from build123d import *

# Parameters (mm, degrees)
CROQUIS1_W              = 72
CROQUIS1_H              = 180
CROQUIS1_R              = 1.6
SALIENTE_EXTRUIR1_DEPTH = 4
CROQUIS2_R              = 3
CORTAR_EXTRUIR1_DEPTH   = 1.65
CROQUIS3_W              = 5
CROQUIS3_H              = 10
SALIENTE_EXTRUIR2_DEPTH = 10
CORTAR_EXTRUIR2_REACH   = 263.951
CROQUIS4_R              = 1.5
CROQUIS4_3_R            = 1.5
CORTAR_EXTRUIR3_DEPTH   = 1.65
REDONDEO2_R             = 10
CORTAR_EXTRUIR4_REACH   = 262.458
CROQUIS6_W              = 11.3
CROQUIS6_H              = 119.12
CORTAR_EXTRUIR5_DEPTH   = 4
REDONDEO3_R             = 3


with BuildPart() as part:
    # Croquis1 → Saliente-Extruir1 (new body)
    with BuildSketch(Plane.XY):
        with Locations((26, 162.773389683)):
            Rectangle(CROQUIS1_W, CROQUIS1_H)
        with Locations((-1.52, 76.973389683)):
            Circle(CROQUIS1_R, mode=Mode.SUBTRACT)
        with Locations((5.52, 83.573389683)):
            Circle(CROQUIS1_R, mode=Mode.SUBTRACT)
        with Locations((-1.52, 241.973389683)):
            Circle(CROQUIS1_R, mode=Mode.SUBTRACT)
        with Locations((5.52, 248.573389683)):
            Circle(CROQUIS1_R, mode=Mode.SUBTRACT)
    extrude(amount=SALIENTE_EXTRUIR1_DEPTH)

    # Croquis2 → Cortar-Extruir1 (cut)
    with BuildSketch(Plane.XY.offset(4)):
        with Locations((-1.52, 76.973389683)):
            Circle(CROQUIS2_R)
        with Locations((5.52, 83.573389683)):
            Circle(CROQUIS2_R)
        with Locations((-1.52, 241.973389683)):
            Circle(CROQUIS2_R)
        with Locations((5.52, 248.573389683)):
            Circle(CROQUIS2_R)
    extrude(amount=-CORTAR_EXTRUIR1_DEPTH, mode=Mode.SUBTRACT)

    # Croquis3 → Saliente-Extruir2 (add)
    with BuildSketch(Plane(origin=(0, 0, 0), x_dir=(-1, 0, 0), z_dir=(0, 0, -1))):
        with Locations((3.5, 125.273389683)):
            Rectangle(CROQUIS3_W, CROQUIS3_H)
        with Locations((3.5, 200.273389683)):
            Rectangle(CROQUIS3_W, CROQUIS3_H)
    extrude(amount=SALIENTE_EXTRUIR2_DEPTH)

    # Croquis4 → Cortar-Extruir2 (cut, up to next)
    with BuildSketch(Plane.ZY.offset(6), mode=Mode.PRIVATE) as cortar_extruir2_sk1:
        with Locations(Location((-5, 125.273389683, 0), (0, 0, 270))):
            Circle(CROQUIS4_R)
    cortar_extruir2_tool1 = extrude(cortar_extruir2_sk1.sketch, amount=-CORTAR_EXTRUIR2_REACH, mode=Mode.PRIVATE) & part.part
    # Croquis4 → Cortar-Extruir2 (cut, up to next)
    with BuildSketch(Plane.ZY.offset(6), mode=Mode.PRIVATE) as cortar_extruir2_sk2:
        with Locations(Location((-5, 200.273389683, 0), (0, 0, 270))):
            Circle(CROQUIS4_R)
    cortar_extruir2_tool2 = extrude(cortar_extruir2_sk2.sketch, amount=-CORTAR_EXTRUIR2_REACH, mode=Mode.PRIVATE) & part.part
    add(cortar_extruir2_tool1.solids().sort_by_distance((-6, 125.27339, -5))[0], mode=Mode.SUBTRACT)
    add(cortar_extruir2_tool2.solids().sort_by_distance((-6, 200.27339, -5))[0], mode=Mode.SUBTRACT)

    # Croquis4<3> → Cortar-Extruir3 (cut)
    # profile 1 of 2: a face of its own
    with BuildSketch(Plane.ZY.offset(6)):
        Polygon((-8.175426481, 200.273389683), (-6.58771324, 197.523389683), (-3.41228676, 197.523389683), (-1.824573519, 200.273389683), (-3.41228676, 203.023389683), (-6.58771324, 203.023389683), align=None)
        with Locations(Location((-5, 200.273389683, 0), (0, 0, 270))):
            Circle(CROQUIS4_3_R, mode=Mode.SUBTRACT)
    # profile 2 of 2: a face of its own
    with BuildSketch(Plane.ZY.offset(6)):
        Polygon((-8.175426481, 125.273389683), (-6.58771324, 122.523389683), (-3.41228676, 122.523389683), (-1.824573519, 125.273389683), (-3.41228676, 128.023389683), (-6.58771324, 128.023389683), align=None)
        with Locations(Location((-5, 125.273389683, 0), (0, 0, 270))):
            Circle(CROQUIS4_3_R, mode=Mode.SUBTRACT)
    extrude(amount=-CORTAR_EXTRUIR3_DEPTH, mode=Mode.SUBTRACT)

    # Redondeo2
    # the kernel refuses this fillet: 10 mm, written as the material it takes off along each edge
    with BuildSketch(Plane(origin=(62, 52.773389683, 4), x_dir=(0, 0, -1), z_dir=(0, 1, 0))) as redondeo2_piece_1:
        with BuildLine():
            CenterArc((10, 8), REDONDEO2_R, 180, 53.130102354)
            Line((0, 8), (-0.2, 8))
            Line((-0.2, 8), (-0.2, 0))
            Line((-0.2, 0), (0, -0.2))
            ThreePointArc((0, -0.2), (2, -0.2), (3.88, -0.16))
            Line((3.88, -0.16), (4, 0))
        make_face()
    extrude(amount=220, mode=Mode.SUBTRACT)

    # Croquis5 → Cortar-Extruir4 (cut, up to next)
    with BuildSketch(Plane(origin=(0, 0, 0), x_dir=(-1, 0, 0), z_dir=(0, 0, -1)), mode=Mode.PRIVATE) as cortar_extruir4_sk1:
        with BuildLine():
            Line((-18.04, 177.143389683), (-18.04, 170.803389683))
            ThreePointArc((-18.04, 170.803389683), (-18.479339828, 169.742729511), (-19.54, 169.303389683))
            Line((-19.54, 169.303389683), (-20.1, 169.303389683))
            ThreePointArc((-20.1, 169.303389683), (-21.160660172, 169.742729511), (-21.6, 170.803389683))
            Line((-21.6, 170.803389683), (-21.6, 177.143389683))
            ThreePointArc((-21.6, 177.143389683), (-21.160660172, 178.204049855), (-20.1, 178.643389683))
            Line((-20.1, 178.643389683), (-19.54, 178.643389683))
            ThreePointArc((-19.54, 178.643389683), (-18.479339828, 178.204049855), (-18.04, 177.143389683))
        make_face()
    cortar_extruir4_tool1 = extrude(cortar_extruir4_sk1.sketch, amount=-CORTAR_EXTRUIR4_REACH, mode=Mode.PRIVATE) & part.part
    # Croquis5 → Cortar-Extruir4 (cut, up to next)
    with BuildSketch(Plane(origin=(0, 0, 0), x_dir=(-1, 0, 0), z_dir=(0, 0, -1)), mode=Mode.PRIVATE) as cortar_extruir4_sk2:
        with BuildLine():
            Line((-18.3, 191.373389683), (-18.3, 185.773389683))
            ThreePointArc((-18.3, 185.773389683), (-18.490380592, 185.313770275), (-18.95, 185.123389683))
            Line((-18.95, 185.123389683), (-20.27019783, 185.123389683))
            ThreePointArc((-20.27019783, 185.123389683), (-20.510915139, 185.169605635), (-20.717401742, 185.301681447))
            Line((-20.717401742, 185.301681447), (-21.397203913, 185.946169218))
            ThreePointArc((-21.397203913, 185.946169218), (-21.547152637, 186.161150502), (-21.6, 186.417877455))
            Line((-21.6, 186.417877455), (-21.6, 188.413389575))
            Line((-21.6, 188.413389575), (-21.6, 190.728901911))
            ThreePointArc((-21.6, 190.728901911), (-21.547152637, 190.985628864), (-21.397203913, 191.200610148))
            Line((-21.397203913, 191.200610148), (-20.717401742, 191.84509792))
            ThreePointArc((-20.717401742, 191.84509792), (-20.510915139, 191.977173731), (-20.27019783, 192.023389683))
            Line((-20.27019783, 192.023389683), (-18.95, 192.023389683))
            ThreePointArc((-18.95, 192.023389683), (-18.490380592, 191.833009091), (-18.3, 191.373389683))
        make_face()
    cortar_extruir4_tool2 = extrude(cortar_extruir4_sk2.sketch, amount=-CORTAR_EXTRUIR4_REACH, mode=Mode.PRIVATE) & part.part
    # Croquis5 → Cortar-Extruir4 (cut, up to next)
    with BuildSketch(Plane(origin=(0, 0, 0), x_dir=(-1, 0, 0), z_dir=(0, 0, -1)), mode=Mode.PRIVATE) as cortar_extruir4_sk3:
        with BuildLine():
            Line((-18.95, 198.523389683), (-20.27019783, 198.523389683))
            ThreePointArc((-20.27019783, 198.523389683), (-20.510915139, 198.569605635), (-20.717401742, 198.701681447))
            Line((-20.717401742, 198.701681447), (-21.397203913, 199.346169218))
            ThreePointArc((-21.397203913, 199.346169218), (-21.547152637, 199.561150502), (-21.6, 199.817877455))
            Line((-21.6, 199.817877455), (-21.6, 201.813389575))
            Line((-21.6, 201.813389575), (-21.6, 204.128901911))
            ThreePointArc((-21.6, 204.128901911), (-21.547152637, 204.385628864), (-21.397203913, 204.600610148))
            Line((-21.397203913, 204.600610148), (-20.717401742, 205.24509792))
            ThreePointArc((-20.717401742, 205.24509792), (-20.510915139, 205.377173731), (-20.27019783, 205.423389683))
            Line((-20.27019783, 205.423389683), (-18.95, 205.423389683))
            ThreePointArc((-18.95, 205.423389683), (-18.490380592, 205.233009091), (-18.3, 204.773389683))
            Line((-18.3, 204.773389683), (-18.3, 199.173389683))
            ThreePointArc((-18.3, 199.173389683), (-18.490380592, 198.713770275), (-18.95, 198.523389683))
        make_face()
    cortar_extruir4_tool3 = extrude(cortar_extruir4_sk3.sketch, amount=-CORTAR_EXTRUIR4_REACH, mode=Mode.PRIVATE) & part.part
    add(cortar_extruir4_tool1.solids().sort_by_distance((19.82, 173.97339, 0))[0], mode=Mode.SUBTRACT)
    add(cortar_extruir4_tool2.solids().sort_by_distance((19.895302, 188.57339, 0))[0], mode=Mode.SUBTRACT)
    add(cortar_extruir4_tool3.solids().sort_by_distance((19.895302, 201.97339, 0))[0], mode=Mode.SUBTRACT)

    # Croquis6 → Cortar-Extruir5 (cut)
    with BuildSketch(Plane.XY.offset(4)):
        with Locations((18.95, 148.863389683)):
            Rectangle(CROQUIS6_W, CROQUIS6_H)
    extrude(amount=-CORTAR_EXTRUIR5_DEPTH, mode=Mode.SUBTRACT)

    # Redondeo3
    redondeo3_edges = [part.edges().sort_by_distance(p)[0] for p in [
        (13.3, 89.303389683, 2),
        (13.3, 208.423389683, 2),
        (24.6, 208.423389683, 2),
        (24.6, 89.303389683, 2),
    ]]
    fillet(redondeo3_edges, radius=REDONDEO3_R)


solid = part.part
Verification items for the finished model (mm, model axes). A direction names the side the tool comes from. Coordinates: 2 decimals unless noted, no trailing zeros. Order: outer loops, then holes, each group sorted by start corner. A loop starts at its lowest first (then second) coordinate and runs counter-clockwise, first axis right, second up.
1. Go/stop test with flat-tipped pins: pin 1 Ø4 at (x, y) = (-1.52, 76.97) entering from -Z; pin 2 Ø3.5 at (x, y) = (-1.52, 241.97) entering from +Z; pin 3 Ø8 at (x, z) = (-1, -3) entering from -Y; pin 4 Ø0.8 at (x, z) = (-5, -5) entering from -Y. Record where each tip stops, or that it passes through.
Results found:
pin 1: stops at z = 0
pin 2: stops at z = 2.35
pin 3: stops at y = 72.77
pin 4: stops at y = 120.27
2. Sectioned sample at A-A, the plane y = 115.5. Record the cut outline in (x, z), and give its area (3 significant figures).
Results found:
outline: (-10, 0) - (13.3, 0) - (13.3, 4) - (-10, 4) - close; (24.6, 0) - (62, 0) arc R10 ccw to (54, 4) - (24.6, 4) - close
area: 233 mm2
3. Scan lines: line 1 (Y direction, x = 5.52, z = 0.9); line 2 (Y direction, x = -1.52, z = 1.7); line 3 (Z direction, x = -2, y = 135). Record each from-to range of solid material in increasing order.
Results found:
line 1: y = 72.77 to 81.97, 85.17 to 246.97, 250.17 to 252.77
line 2: y = 72.77 to 75.37, 78.57 to 240.37, 243.57 to 252.77
line 3: z = 0 to 4
4. Sectioned sample at D-D, the plane x = 48.5. Record the cut outline in (y, z), and give its area (3 significant figures).
Results found:
outline: (72.77, 0) - (252.77, 0) - (252.77, 4) - (72.77, 4) - close
area: 720 mm2
5. Set-up check for faces 5 (the face through (-3, 125, -10)), 6 (the face through (7, 247, 2.35)), 7 (the face through (-3, 195.273, -5)), 8 (the face through (14.202, 207.568, 1.972)), 9 (the face through (-3, 205.273, -5)): record each of +Z, -Z, +X, -X, +Y, -Y from which the full face is reachable in a straight line by a thin tool's end or side.
Results found:
face 5: -Z, +X, -X, +Y, -Y
face 6: +Z
face 7: -Z, +X, -X
face 8: +Z, -Z
face 9: -Z, +X, -X, +Y
6. Sectioned sample at C-C, the plane y = 228.5. Record the cut outline in (x, z), and give its area (3 significant figures).
Results found:
outline: (-10, 0) - (62, 0) arc R10 ccw to (54, 4) - (-10, 4) - close
area: 278 mm2
7. Release check for a two-part mould opening along Z. For faces 1 (the face through (58.414, 161.513, 2.973)), 2 (the face through (-2.698, 123.843, -4.549)), 3 (the face through (4.87, 80.645, 3.187)), 4 (the face through (-4.35, 127, -4)) record: +Z half, -Z half, draft (parallel to the pull), parting line (faces both ways), or undercut.
Results found:
face 1: +Z half
face 2: undercut
face 3: draft
face 4: undercut
8. Sectioned sample at B-B, the plane x = 5.52. Record the cut outline in (y, z).
Results found:
outline: (72.77, 0) - (81.97, 0) - (81.97, 2.35) - (80.57, 2.35) - (80.57, 4) - (72.77, 4) - close; (85.17, 0) - (246.97, 0) - (246.97, 2.35) - (245.57, 2.35) - (245.57, 4) - (86.57, 4) - (86.57, 2.35) - (85.17, 2.35) - close; (250.17, 0) - (252.77, 0) - (252.77, 4) - (251.57, 4) - (251.57, 2.35) - (250.17, 2.35) - close
